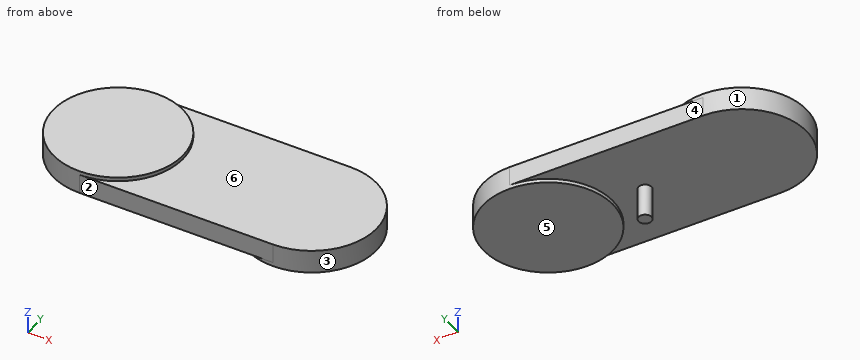
from build123d import *

# Parameters (mm, degrees)
SKETCH_1_W      = 150
SKETCH_1_H      = 100
EXTRUDE_1_DEPTH = 15
EXTRUDE_4_DEPTH = 15
EXTRUDE_6_DEPTH = 18
EXTRUDE_START   = -3
EXTRUDE_7_DEPTH = 3
SKETCH_1_17_R   = 5
EXTRUDE_8_DEPTH = 25


with BuildPart() as part:
    # Sketch 1 → Extrude 1 (new body)
    with BuildSketch(Plane.XY):
        with Locations((-75, 50)):
            Rectangle(SKETCH_1_W, SKETCH_1_H)
    extrude(amount=EXTRUDE_1_DEPTH)

    # Sketch 1_10 → Extrude 4 (add)
    with BuildSketch(Plane.XY):
        with BuildLine():
            ThreePointArc((50, 50), (35.355339059, 85.355339059), (0, 100))
            Line((0, 100), (0, 75))
            ThreePointArc((0, 75), (17.67766953, 67.67766953), (25, 50))
            ThreePointArc((25, 50), (17.67766953, 32.32233047), (0, 25))
            Line((0, 25), (0, 0))
            ThreePointArc((0, 0), (35.355339059, 14.644660941), (50, 50))
        make_face()
        with BuildLine():
            ThreePointArc((25, 50), (17.67766953, 67.67766953), (0, 75))
            Line((0, 75), (0, 50))
            Line((0, 50), (0, 25))
            ThreePointArc((0, 25), (17.67766953, 32.32233047), (25, 50))
        make_face()
        with BuildLine():
            Line((-150, 25), (-150, 50))
            Line((-150, 50), (-150, 75))
            ThreePointArc((-150, 75), (-175, 50), (-150, 25))
        make_face()
        with BuildLine():
            Line((-150, 75), (-150, 100))
            ThreePointArc((-150, 100), (-200, 50), (-150, 0))
            Line((-150, 0), (-150, 25))
            ThreePointArc((-150, 25), (-175, 50), (-150, 75))
        make_face()
    extrude(amount=EXTRUDE_4_DEPTH)

    # Sketch 1_14 → Extrude 6 (add)
    with BuildSketch(Plane.XY):
        with BuildLine():
            ThreePointArc((-150, 0), (-114.644660941, 14.644660941), (-100, 50))
            Line((-100, 50), (-125, 50))
            ThreePointArc((-125, 50), (-132.32233047, 32.32233047), (-150, 25))
            Line((-150, 25), (-150, 0))
        make_face()
        with BuildLine():
            Line((-125, 50), (-100, 50))
            ThreePointArc((-100, 50), (-114.644660941, 85.355339059), (-150, 100))
            Line((-150, 100), (-150, 75))
            ThreePointArc((-150, 75), (-132.32233047, 67.67766953), (-125, 50))
        make_face()
        with BuildLine():
            Line((-150, 75), (-150, 100))
            ThreePointArc((-150, 100), (-200, 50), (-150, 0))
            Line((-150, 0), (-150, 25))
            ThreePointArc((-150, 25), (-175, 50), (-150, 75))
        make_face()
        with BuildLine():
            ThreePointArc((-150, 25), (-132.32233047, 32.32233047), (-125, 50))
            Line((-125, 50), (-150, 50))
            Line((-150, 50), (-150, 25))
        make_face()
        with BuildLine():
            Line((-150, 50), (-125, 50))
            ThreePointArc((-125, 50), (-132.32233047, 67.67766953), (-150, 75))
            Line((-150, 75), (-150, 50))
        make_face()
        with BuildLine():
            Line((-150, 25), (-150, 50))
            Line((-150, 50), (-150, 75))
            ThreePointArc((-150, 75), (-175, 50), (-150, 25))
        make_face()
    extrude(amount=EXTRUDE_6_DEPTH)

    # Sketch 1_16 → Extrude 7 (add)
    with BuildSketch(Plane.XY.offset(EXTRUDE_START)):
        with BuildLine():
            ThreePointArc((50, 50), (35.355339059, 85.355339059), (0, 100))
            Line((0, 100), (0, 75))
            ThreePointArc((0, 75), (17.67766953, 67.67766953), (25, 50))
            ThreePointArc((25, 50), (17.67766953, 32.32233047), (0, 25))
            Line((0, 25), (0, 0))
            ThreePointArc((0, 0), (35.355339059, 14.644660941), (50, 50))
        make_face()
        with BuildLine():
            Line((0, 75), (0, 100))
            ThreePointArc((0, 100), (-35.355339059, 85.355339059), (-50, 50))
            Line((-50, 50), (-25, 50))
            ThreePointArc((-25, 50), (-17.67766953, 67.67766953), (0, 75))
        make_face()
        with BuildLine():
            ThreePointArc((-50, 50), (-35.355339059, 14.644660941), (0, 0))
            Line((0, 0), (0, 25))
            ThreePointArc((0, 25), (-17.67766953, 32.32233047), (-25, 50))
            Line((-25, 50), (-50, 50))
        make_face()
        with BuildLine():
            Line((0, 50), (0, 75))
            ThreePointArc((0, 75), (-17.67766953, 67.67766953), (-25, 50))
            Line((-25, 50), (0, 50))
        make_face()
        with BuildLine():
            ThreePointArc((-25, 50), (-17.67766953, 32.32233047), (0, 25))
            Line((0, 25), (0, 50))
            Line((0, 50), (-25, 50))
        make_face()
        with BuildLine():
            ThreePointArc((25, 50), (17.67766953, 67.67766953), (0, 75))
            Line((0, 75), (0, 50))
            Line((0, 50), (0, 25))
            ThreePointArc((0, 25), (17.67766953, 32.32233047), (25, 50))
        make_face()
    extrude(amount=EXTRUDE_7_DEPTH)

    # Sketch 1_17 → Extrude 8 (add)
    with BuildSketch(Plane.XY):
        with Locations((-75, 50)):
            Circle(SKETCH_1_17_R)
    extrude(amount=-EXTRUDE_8_DEPTH)


solid = part.part
Can you work these out from the model? Positions are in its coordinate system, mm. Face numbers are marked on the shaded views. A direction names the side the tool comes from. Round coordinates to 2 decimals unless told otherwise and drop trailing zeros. Loops run counter-clockwise (first coordinate to the right, second up) from the corner with the lowest first, then second, coordinate; pieces in that order, holes last. Notation, with made-up numbers: (-26.5, 51.5) - (17.5, 51.5) arc R21 cw to (17.5, 59.5) - close; hole circle Ø5 at (15.5, 12.25). An arc over 180 degrees is marked (long way). Answer in a Markdown table with one row per item. Add a question column.
Q1. I want a section at C-C on z = -14.5. List the corners of the cut face in (x, y) for me.
Q2. I want a section at D-D on y = 61. List the corners of the cut face in (x, z) for me (3 decimals), and give its area (3 significant figures).
Q3. Which directions (+Z, -Z, +X, -X, +Y, -Y) give clear straight access to the entire face, cutting with the end or side of a thin tool? Please do the marked faces 1, 2 and 3.
Q4. I want a section at A-A on x = -75. List the corners of the cut face in (y, z) for me, and give its area (3 significant figures).
Q5. I want a section at B-B on y = 50. List the corners of the cut face in (x, z) for me, and give its area (3 significant figures).
Q6. We'd pull the mould along Z, two halves only. Please class the marked faces 4, 5 and 6: pulls with the +Z half, pulls with the -Z half, needs draft (parallel to the pull), parting line crosses it, or undercut.
Q7. I need wall thicknesses on L1, parallel to Z at x = -157, y = 74; L2, parallel to Z at x = -10, y = 36.5; L3, parallel to X at y = 51.5, z = 9. Which ranges of each line are inside material? Lowest first, please.
Q8. For pin 1 Ø12 at (x, y) = (-69.5, 83) entering from +Z; pin 2 Ø5 at (y, z) = (60.5, 0) entering from +X; pin 3 Ø2 at (x, y) = (-46.5, 68.5) entering from -Z, each with a flat end and sliding along its axis, tell me the tip position at first contact or that it passes through.
A:
| question | item | result |
|---|---|---|
| 1 | outline | circle Ø10 at (-75, 50) |
| 2 | outline | (-198.775, 0) - (-48.775, 0) - (-48.775, -3) - (48.775, -3) - (48.775, 15) - (-101.225, 15) - (-101.225, 18) - (-198.775, 18) - close |
| 2 | area | 4,300 mm^2 |
| 3 | face 1 | +Z |
| 3 | face 2 | +Z, -Z, +X, -X, -Y |
| 3 | face 3 | -Z |
| 4 | outline | (0, 0) - (45, 0) - (45, -25) - (55, -25) - (55, 0) - (100, 0) - (100, 15) - (0, 15) - close |
| 4 | area | 1,750 mm^2 |
| 5 | outline | (-200, 0) - (-80, 0) - (-80, -25) - (-70, -25) - (-70, 0) - (-50, 0) - (-50, -3) - (50, -3) - (50, 15) - (-100, 15) - (-100, 18) - (-200, 18) - close |
| 5 | area | 4,600 mm^2 |
| 6 | face 4 | needs draft |
| 6 | face 5 | pulls with the -Z half |
| 6 | face 6 | pulls with the +Z half |
| 7 | L1 | 0 to 18 |
| 7 | L2 | -3 to 15 |
| 7 | L3 | -199.98 to 49.98 |
| 8 | pin 1 | z = 15 |
| 8 | pin 2 | x = 49.36 |
| 8 | pin 3 | z = -3 |
